Build history of the part. All positions in model axes, mm. A direction names the side the tool comes from. Round coordinates to 2 decimals unless told otherwise and drop trailing zeros. Order: outer loops, then holes, each group sorted by start corner. A loop starts at its lowest first (then second) coordinate and runs counter-clockwise, first axis right, second up. Notation, with made-up numbers: (67, 82.5) -> (125, 82.5) arc R26 ccw to (125, 116.5) -> close; hole circle Ø2 at (51.25, 51.25). An arc over 180 degrees is marked (long way). Write item = value, one per line.
from build123d import *

# Parameters (mm, degrees)
SKETCH2_R           = 110
BOSS_EXTRUDE2_DEPTH = 10
SKETCH3_R           = 2
CUT_EXTRUDE1_DEPTH  = 10
SKETCH4_R           = 5
CUT_EXTRUDE2_DEPTH  = 6
SKETCH5_R           = 2
CUT_EXTRUDE3_DEPTH  = 156.884572681
CUT_EXTRUDE9_START  = -6
SKETCH7_R           = 4.5
SKETCH7_R_2         = 2
CUT_EXTRUDE9_DEPTH  = 6
SKETCH8_R           = 4.5
CUT_EXTRUDE10_DEPTH = 6


with BuildPart() as part:
    # Sketch2 → Boss-Extrude2 (new body)
    with BuildSketch(Plane(origin=(0, 0, 0), x_dir=(1, 0, 0), z_dir=(0, 1, 0))):
        with Locations(Location((0, 0, 0), (0, 0, 270))):
            Circle(SKETCH2_R)
    extrude(amount=BOSS_EXTRUDE2_DEPTH)

    # Sketch3 → Cut-Extrude1 (cut)
    with BuildSketch(Plane(origin=(0, 10, 0), x_dir=(1, 0, 0), z_dir=(0, 1, 0))):
        with Locations(Location((0, 95, 0), (0, 0, 270))):
            Circle(SKETCH3_R)
        with Locations(Location((67.175144213, 67.175144213, 0), (0, 0, 270))):
            Circle(SKETCH3_R)
        with Locations(Location((95, 0, 0), (0, 0, 270))):
            Circle(SKETCH3_R)
        with Locations(Location((67.175144213, -67.175144213, 0), (0, 0, 270))):
            Circle(SKETCH3_R)
        with Locations(Location((0, -95, 0), (0, 0, 270))):
            Circle(SKETCH3_R)
        with Locations(Location((-67.175144213, -67.175144213, 0), (0, 0, 270))):
            Circle(SKETCH3_R)
        with Locations(Location((-95, 0, 0), (0, 0, 270))):
            Circle(SKETCH3_R)
        with Locations(Location((-67.175144213, 67.175144213, 0), (0, 0, 270))):
            Circle(SKETCH3_R)
    extrude(amount=-CUT_EXTRUDE1_DEPTH, mode=Mode.SUBTRACT)

    # Sketch4 → Cut-Extrude2 (cut)
    with BuildSketch(Plane(origin=(0, 0, 0), x_dir=(1, 0, 0), z_dir=(0, 1, 0))):
        with Locations(Location((0, 95, 0), (0, 0, 270))):
            Circle(SKETCH4_R)
        with Locations(Location((67.175144213, 67.175144213, 0), (0, 0, 270))):
            Circle(SKETCH4_R)
        with Locations(Location((95, 0, 0), (0, 0, 270))):
            Circle(SKETCH4_R)
        with Locations(Location((67.175144213, -67.175144213, 0), (0, 0, 270))):
            Circle(SKETCH4_R)
        with Locations(Location((0, -95, 0), (0, 0, 270))):
            Circle(SKETCH4_R)
        with Locations(Location((-67.175144213, -67.175144213, 0), (0, 0, 270))):
            Circle(SKETCH4_R)
        with Locations(Location((-95, 0, 0), (0, 0, 270))):
            Circle(SKETCH4_R)
        with Locations(Location((-67.175144213, 67.175144213, 0), (0, 0, 270))):
            Circle(SKETCH4_R)
    extrude(amount=CUT_EXTRUDE2_DEPTH, mode=Mode.SUBTRACT)

    # Sketch5 → Cut-Extrude3 (cut, through all)
    with BuildSketch(Plane(origin=(0, 10, 0), x_dir=(1, 0, 0), z_dir=(0, 1, 0))):
        with Locations(Location((5, 14.5, 0), (0, 0, 270))):
            Circle(SKETCH5_R)
        with Locations(Location((-5, 14.5, 0), (0, 0, 270))):
            Circle(SKETCH5_R)
        with Locations(Location((5, -35, 0), (0, 0, 270))):
            Circle(SKETCH5_R)
        with Locations(Location((-5, -35, 0), (0, 0, 270))):
            Circle(SKETCH5_R)
    extrude(amount=-CUT_EXTRUDE3_DEPTH, mode=Mode.SUBTRACT)

    # Sketch7 → Cut-Extrude9 (cut)
    # profile 1 of 2: a face of its own
    with BuildSketch(Plane.XZ.offset(CUT_EXTRUDE9_START)):
        with Locations(Location((5, -14.5, 0), (0, 0, 270))):
            Circle(SKETCH7_R)
        with Locations(Location((5, -14.5, 0), (0, 0, 90))):
            Circle(SKETCH7_R_2, mode=Mode.SUBTRACT)
    # profile 2 of 2: a face of its own
    with BuildSketch(Plane.XZ.offset(CUT_EXTRUDE9_START)):
        with Locations(Location((-5, -14.5, 0), (0, 0, 270))):
            Circle(SKETCH7_R)
        with Locations(Location((-5, -14.5, 0), (0, 0, 90))):
            Circle(SKETCH7_R_2, mode=Mode.SUBTRACT)
    extrude(amount=CUT_EXTRUDE9_DEPTH, mode=Mode.SUBTRACT)

    # Sketch8 → Cut-Extrude10 (cut)
    with BuildSketch(Plane.XZ):
        with Locations(Location((5, 35, 0), (0, 0, 270))):
            Circle(SKETCH8_R)
        with Locations(Location((-5, 35, 0), (0, 0, 270))):
            Circle(SKETCH8_R)
    extrude(amount=-CUT_EXTRUDE10_DEPTH, mode=Mode.SUBTRACT)


solid = part.part
Q1. Mould opens along Z. For faces 1 (the face through (-62.959, 2.958, -64.487)), 2 (the face through (2, 10, -2)), 3 (the face through (65.26, 2.958, -62.556)) say: released by +Z, released by -Z, zero draft, split by the parting line, or undercut.
Check values:
face_1 = undercut
face_2 = zero draft
face_3 = undercut
Q2. Cut at C-C, the plane z = -59. List the corners of the cut face in (x, y).
Check values:
outline = (-92.84, 0) -> (92.84, 0) -> (92.84, 10) -> (-92.84, 10) -> close
Q3. Cut at A-A, the plane y = 2.5. Give the number of separate pieces and of enclosed holes in the cut face, and give its area (3 significant figures).
Check values:
separate_pieces = 1
enclosed_holes = 12
area = 37,100 mm²
Q4. Cut at B-B, the plane x = 38.5. List the corners of the cut face in (y, z).
Check values:
outline = (0, -103.04) -> (10, -103.04) -> (10, 103.04) -> (0, 103.04) -> close
Q5. Flat gauge pins, fed straight in: pin 1 (3 mm diameter, centred on x = -94, z = -1, fed in from -Y); pin 2 (2.5 mm diameter, centred on x = -5, z = 35, fed in from +Y); pin 3 (4 mm diameter, centred on x = -82.5, y = 2.5, fed in from -Z) (3 decimals); pin 4 (1 mm diameter, centred on x = 2.5, y = 1.5, fed in from -Z). Where does each tip first touch, or does it go through?
Check values:
pin_1 = 6
pin_2 = through
pin_3 = -74.965
pin_4 = -109.98
Q6. Probe probe 1 along Z at (x, y) = (68, 0.5); probe 2 along Z at (x, y) = (-63, 1.25); probe 3 along X at (y, z) = (1.5, 38). List the from-to ranges inside material, lowest first.
Check values:
probe_1 = -86.46 to -72.11, -62.24 to 62.24, 72.11 to 86.46
probe_2 = -90.17 to -69.93, -64.42 to 64.42, 69.93 to 90.17
probe_3 = -103.23 to -8.35, -1.65 to 1.65, 8.35 to 103.23
Q7. Which spindle directions (+Z, -Z, +X, -X, +Y, -Y) get a long thin tool onto all of the face, cutting with end or side? Do faces 4 (the face through (-2.2, 6, 94.9)), 5 (the face through (2, 0, -2)). Say none if no direction does.
Check values:
face_4 = -Y
face_5 = +Z, -Z, +X, -X, -Y
